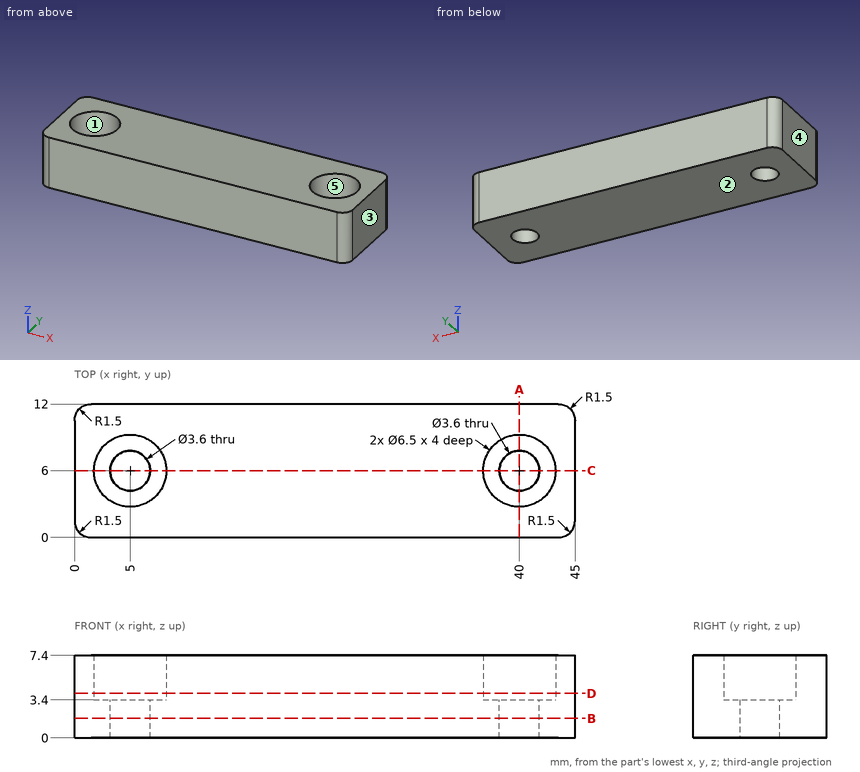
The figure shows three views and two pictorial views of one solid part (mm, origin at its lowest corner). Answer the questions. A direction names the side the tool comes from. Coordinates: 2 decimals unless noted, no trailing zeros. Loops run counter-clockwise (first coordinate to the right, second up) from the corner with the lowest first, then second, coordinate; pieces in that order, holes last. Notation, with made-up numbers: (-17.5, 49.5) -> (19.5, 49.5) arc R28 ccw to (19.5, 86.5) -> close; hole circle Ø6 at (10, 73). An arc over 180 degrees is marked (long way). Return JSON: item names as keys, results as strings. Group by question number.
(1) A cutting plane is placed at D-D on z = 4. Write down the section's boundary in (x, y), and give its area (3 significant figures).
(2) A cutting plane is placed at A-A on x = 40. Write down the section's boundary in (y, z).
(3) Given pin 1 Ø4 at (x, y) = (40, 6) entering from +Z, flat-ended and moving along its own axis, determine where the tip first touches the part or whether it passes through.
(4) A cutting plane is placed at C-C on y = 6. Write down the section's boundary in (x, z).
(5) Determine the mould class of the marked faces 3, 4 and 5 for opening direction X: released by +X, released by -X, zero draft, split by the parting line, or undercut.
(6) Which of the six approach directions +Z, -Z, +X, -X, +Y, -Y give full straight-line access (tool end or side, diameter ignored) to the marked faces 1 and 2?
(7) A cutting plane is placed at B-B on z = 1.75. Write down the section's boundary in (x, y), and give its area (3 significant figures).
(8) Find the intervals of material crossed by probe 1 along X at (y, z) = (6, 6.4); probe 2 along Y at (x, z) = (5, 6.15); probe 3 along X at (y, z) = (4.5, 3.5), in increasing order. Write a range as from..to.
The answers:
{
 "1": {"outline": "(0, 1.5) arc R1.5 ccw to (1.5, 0) -> (43.5, 0) arc R1.5 ccw to (45, 1.5) -> (45, 10.5) arc R1.5 ccw to (43.5, 12) -> (1.5, 12) arc R1.5 ccw to (0, 10.5) -> close; hole circle Ø6.5 at (5, 6); hole circle Ø6.5 at (40, 6)", "area": "472 mm^2"},
 "2": {"outline": "(0, 0) -> (4.2, 0) -> (4.2, 3.4) -> (2.75, 3.4) -> (2.75, 7.4) -> (0, 7.4) -> close; (7.8, 0) -> (12, 0) -> (12, 7.4) -> (9.25, 7.4) -> (9.25, 3.4) -> (7.8, 3.4) -> close"},
 "3": {"pin 1": "stops at z = 3.4"},
 "4": {"outline": "(0, 0) -> (3.2, 0) -> (3.2, 3.4) -> (1.75, 3.4) -> (1.75, 7.4) -> (0, 7.4) -> close; (6.8, 0) -> (38.2, 0) -> (38.2, 3.4) -> (36.75, 3.4) -> (36.75, 7.4) -> (8.25, 7.4) -> (8.25, 3.4) -> (6.8, 3.4) -> close; (41.8, 0) -> (45, 0) -> (45, 7.4) -> (43.25, 7.4) -> (43.25, 3.4) -> (41.8, 3.4) -> close"},
 "5": {"face 3": "released by +X", "face 4": "released by -X", "face 5": "undercut"},
 "6": {"face 1": "+Z", "face 2": "-Z, +X, -X, +Y, -Y"},
 "7": {"outline": "(0, 1.5) arc R1.5 ccw to (1.5, 0) -> (43.5, 0) arc R1.5 ccw to (45, 1.5) -> (45, 10.5) arc R1.5 ccw to (43.5, 12) -> (1.5, 12) arc R1.5 ccw to (0, 10.5) -> close; hole circle Ø3.6 at (5, 6); hole circle Ø3.6 at (40, 6)", "area": "518 mm^2"},
 "8": {"probe 1": "x = 0..1.75, 8.25..36.75, 43.25..45", "probe 2": "y = 0..2.75, 9.25..12", "probe 3": "x = 0..2.12, 7.88..37.12, 42.88..45"}
}
